For this review, take the finished solid that the model builds, in its own axes (mm). Face numbers are marked on the shaded views. A direction names the side the tool comes from. Coordinates: 2 decimals unless noted, no trailing zeros. Loops run counter-clockwise (first coordinate to the right, second up) from the corner with the lowest first, then second, coordinate; pieces in that order, holes last. Notation, with made-up numbers: M 53,-27.5 L 105,-27.5 A28 ccw 105,6.5 Z; hole C 77.5,9.5 d6. An arc over 180 degrees is marked long. Use one line per item in the form item = value.
```python
from build123d import *

# Parameters (mm, degrees)
F0_W     = 1797.05
F0_H     = 901.7
F1_DEPTH = 50.8
F2_W     = 152.4
F2_H     = 50.8
F5_W     = 50.8
F5_H     = 152.4


with BuildPart() as f1:
    # F0 (on Top) → F1 (new body)
    with BuildSketch(Plane.XY):
        Rectangle(F0_W, F0_H)
    extrude(amount=F1_DEPTH)

    # F4: sweep along a path in F3
    with BuildLine(Plane.XZ) as f4_path:
        Line((542.925, 0), (542.925, -635))
        Line((542.925, -635), (-542.925, -635))
        Line((-542.925, -635), (-542.925, 0))
    # F2 (on face) → F4 (sweep)
    with BuildSketch(Plane(origin=(0, 0, 0), x_dir=(1, 0, 0), z_dir=(0, 0, -1))):
        with Locations((542.925, 0)):
            Rectangle(F2_W, F2_H)
    sweep(path=f4_path.line, transition=Transition.RIGHT)

    # F7: sweep along a path in F6
    with BuildLine(Plane.YZ) as f7_path:
        Line((-276.225, 0), (-276.225, -635))
        Line((-276.225, -635), (276.225, -635))
        Line((276.225, -635), (276.225, 0))
    # F5 (on face) → F7 (sweep)
    with BuildSketch(Plane(origin=(0, 0, 0), x_dir=(1, 0, 0), z_dir=(0, 0, -1))):
        with Locations((0, 276.225)):
            Rectangle(F5_W, F5_H)
    sweep(path=f7_path.line, transition=Transition.RIGHT)


solid = f1.part
```
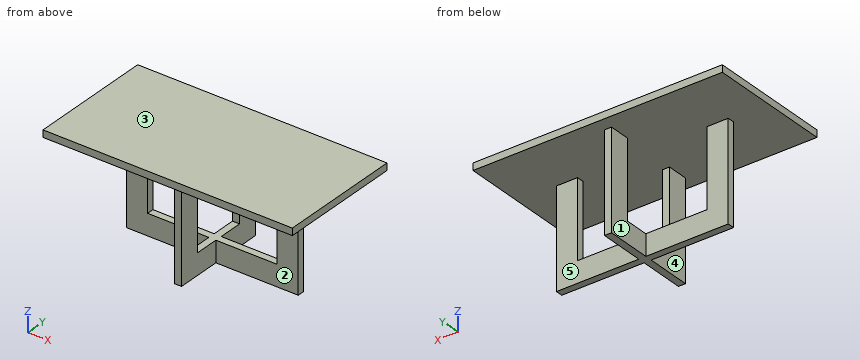
1. Consider section D-D on y = -219. Write out the cut boundary in (x, z) (3 decimals), plus the area to 3 significant figures.
Computed values:
outline = M -898.525,0 L -25.4,0 L -25.4,-711.2 L 25.4,-711.2 L 25.4,0 L 898.525,0 L 898.525,50.8 L -898.525,50.8 Z
area = 127,000 mm2
2. For pin 1 Ø12 at (x, z) = (514.5, -290) entering from -Y; pin 2 Ø3 at (y, z) = (-256.5, -303) entering from -X; pin 3 Ø5 at (x, y) = (-497.5, -254.5) entering from -Z, all flat-tipped, find the tip position at first contact; note any pin that passes through.
Computed values:
pin_1 = -25.4
pin_2 = -25.4
pin_3 = 0
3. Tool access review of the marked faces 1, 2, 3, 4 and 5: name each direction out of +Z, -Z, +X, -X, +Y, -Y from which nothing blocks a thin tool from reaching the whole face with its end or side.
Computed values:
face_1 = -Z, -X, +Y
face_2 = -Z, +X, -Y
face_3 = +Z, +X, -X, +Y, -Y
face_4 = -Z, -X, -Y
face_5 = -Z, +X, +Y
4. Consider section C-C on y = -94. Write out the cut boundary in (x, z) (3 decimals), plus the area to 3 significant figures.
Computed values:
outline = M -898.525,0 L 898.525,0 L 898.525,50.8 L -898.525,50.8 Z; M -25.4,-711.2 L 25.4,-711.2 L 25.4,-558.8 L -25.4,-558.8 Z
area = 99,000 mm2
5. Consider section B-B on z = -295. Write out the cut boundary in (x, y) (3 decimals).
Computed values:
outline = M -619.125,-25.4 L -466.725,-25.4 L -466.725,25.4 L -619.125,25.4 Z; M -25.4,-352.425 L 25.4,-352.425 L 25.4,-200.025 L -25.4,-200.025 Z; M -25.4,200.025 L 25.4,200.025 L 25.4,352.425 L -25.4,352.425 Z; M 466.725,-25.4 L 619.125,-25.4 L 619.125,25.4 L 466.725,25.4 Z
6. Consider section A-A on x = -225. Write out the cut boundary in (y, z), plus the area to 3 significant figures.
Computed values:
outline = M -450.85,0 L 450.85,0 L 450.85,50.8 L -450.85,50.8 Z; M -25.4,-711.2 L 25.4,-711.2 L 25.4,-558.8 L -25.4,-558.8 Z
area = 53,500 mm2
7. Wall thickness on line 1 along Y through (x, z) = (-19, -272.5) (3 decimals); line 2 along Z through (x, y) = (215, 323); line 3 along X through (y, z) = (55.5, -679): over which ranges is each line inside the solid? List them lowest first. Write a range as from..to.
Computed values:
line_1 = -352.425..-200.025, 200.025..352.425
line_2 = 0..50.8
line_3 = -25.4..25.4
